Input: part model. Units: mm. Frame: model coordinates. Face numbers are marked on the shaded views. A direction names the side the tool comes from. Round coordinates to 2 decimals unless told otherwise and drop trailing zeros. Write each loop counter-clockwise with the first axis right and the second up, starting at its lowest first coordinate (ties: lowest second). Pieces come first, ordered by that corner, then holes. Notation, with made-up numbers: (9.25, 17) - (60.25, 17) arc R22 ccw to (60.25, 27) - close; hole circle Ø7 at (-7.5, -11.5). An arc over 180 degrees is marked (long way). Use one line per item in the form item = value.
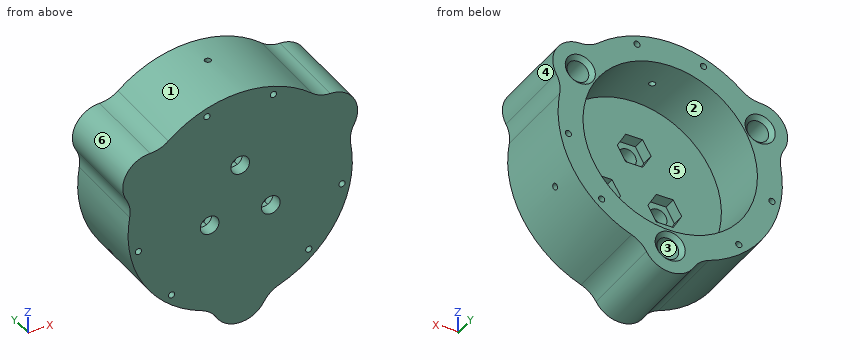
```python
from build123d import *

# Parameters (mm, degrees)
SKETCH_1_R               = 2.625
SKETCH_1_R_2             = 21
EXTRUDE_1_DEPTH          = 15
EXTRUDE_START            = 6
EXTRUDE_2_DEPTH          = 6
FILLET_1_R               = 7
CHAMFER_1_SIZE           = 1
SKETCH_4_R               = 2.25
CUT_EXTRUDE_1_DEPTH      = 48.335527685
CUT_EXTRUDE_2_DEPTH      = 3
SKETCH_6_R               = 0.75
CUT_EXTRUDE_3_DEPTH      = 48.335527685
SKETCH_7_R               = 0.75
CUT_EXTRUDE_4_DEPTH      = 45.996135167
PATTERN_CIRCULAR_1_COUNT = 3


with BuildPart() as part:
    # Эскиз1 → Бобышка-Вытянуть1 (new body)
    with BuildSketch(Plane(origin=(0, 0, 0), x_dir=(1, 0, 0), z_dir=(0, 1, 0))):
        with BuildLine():
            ThreePointArc((25.949265582, -7.458928593), (23.382685902, 13.5), (6.515011145, 26.2021875))
            ThreePointArc((6.515011145, 26.2021875), (0, 31.625), (-6.515011145, 26.2021875))
            ThreePointArc((-6.515011145, 26.2021875), (-23.382685902, 13.5), (-25.949265582, -7.458928593))
            ThreePointArc((-25.949265582, -7.458928593), (-27.388053395, -15.8125), (-19.434254437, -18.743258907))
            ThreePointArc((-19.434254437, -18.743258907), (0, -27), (19.434254437, -18.743258907))
            ThreePointArc((19.434254437, -18.743258907), (27.388053395, -15.8125), (25.949265582, -7.458928593))
        make_face()
        with Locations(Location((0, 25, 0), (0, 0, 270))):
            Circle(SKETCH_1_R, mode=Mode.SUBTRACT)
        with Locations(Location((0, 0, 0), (0, 0, 270))):
            Circle(SKETCH_1_R_2, mode=Mode.SUBTRACT)
        with Locations(Location((-21.650635095, -12.5, 0), (0, 0, 270))):
            Circle(SKETCH_1_R, mode=Mode.SUBTRACT)
        with Locations(Location((21.650635095, -12.5, 0), (0, 0, 270))):
            Circle(SKETCH_1_R, mode=Mode.SUBTRACT)
    extrude(amount=EXTRUDE_1_DEPTH)

    # Эскиз2 → Бобышка-Вытянуть2 (add)
    with BuildSketch(Plane.XZ.offset(EXTRUDE_START)):
        with BuildLine():
            ThreePointArc((25.949265582, 7.458928593), (27.388053395, 15.8125), (19.434254437, 18.743258907))
            ThreePointArc((19.434254437, 18.743258907), (0, 27), (-19.434254437, 18.743258907))
            ThreePointArc((-19.434254437, 18.743258907), (-27.388053395, 15.8125), (-25.949265582, 7.458928593))
            ThreePointArc((-25.949265582, 7.458928593), (-23.382685902, -13.5), (-6.515011145, -26.2021875))
            ThreePointArc((-6.515011145, -26.2021875), (0, -31.625), (6.515011145, -26.2021875))
            ThreePointArc((6.515011145, -26.2021875), (23.382685902, -13.5), (25.949265582, 7.458928593))
        make_face()
    extrude(amount=-EXTRUDE_2_DEPTH)

    # Скругление1
    fillet_1_edges = [part.edges().sort_by_distance(p)[0] for p in [
        (19.434254437, 4.5, 18.743258907),
        (-19.434254437, 4.5, 18.743258907),
        (-25.949265582, 4.5, 7.458928593),
        (-6.515011145, 4.5, -26.2021875),
        (6.515011145, 4.5, -26.2021875),
        (25.949265582, 4.5, 7.458928593),
    ]]
    fillet(fillet_1_edges, radius=FILLET_1_R)

    # Фаска1
    chamfer_1_edges = [part.edges().sort_by_distance(p)[0] for p in [
        (21.650635095, 15, 9.875),
        (0, 15, -27.625),
        (-21.650635095, 15, 9.875),
    ]]
    chamfer(chamfer_1_edges, length=CHAMFER_1_SIZE)

    # Эскиз4 → Вырез-Вытянуть1 (cut, through all)
    with BuildSketch(Plane.XZ.offset(6)):
        with Locations(Location((0, 8.5, 0), (0, 0, 270))):
            Circle(SKETCH_4_R)
        with Locations(Location((7.361215932, -4.25, 0), (0, 0, 270))):
            Circle(SKETCH_4_R)
        with Locations(Location((-7.361215932, -4.25, 0), (0, 0, 270))):
            Circle(SKETCH_4_R)
    extrude(amount=-CUT_EXTRUDE_1_DEPTH, mode=Mode.SUBTRACT)

    # Эскиз5 → Вырез-Вытянуть2 (cut)
    with BuildSketch(Plane(origin=(0, 0, 0), x_dir=(1, 0, 0), z_dir=(0, 1, 0))):
        Polygon((2.035159699, -12.025), (4.070319398, -8.5), (2.035159699, -4.975), (-2.035159699, -4.975), (-4.070319398, -8.5), (-2.035159699, -12.025), align=None)
        Polygon((5.326056233, 0.725), (9.396375631, 0.725), (11.43153533, 4.25), (9.396375631, 7.775), (5.326056233, 7.775), (3.290896534, 4.25), align=None)
        Polygon((-11.43153533, 4.25), (-9.396375631, 0.725), (-5.326056233, 0.725), (-3.290896534, 4.25), (-5.326056233, 7.775), (-9.396375631, 7.775), align=None)
    extrude(amount=-CUT_EXTRUDE_2_DEPTH, mode=Mode.SUBTRACT)

    # Эскиз6 → Вырез-Вытянуть3 (cut, through all)
    with BuildSketch(Plane(origin=(0, 15, 0), x_dir=(1, 0, 0), z_dir=(0, 1, 0))):
        with Locations(Location((-8, -23.685438565, 0), (0, 0, 270))):
            Circle(SKETCH_6_R)
        with Locations(Location((8, -23.685438565, 0), (0, 0, 270))):
            Circle(SKETCH_6_R)
        with Locations(Location((-16.512191497, 18.770922513, 0), (0, 0, 270))):
            Circle(SKETCH_6_R)
        with Locations(Location((-24.512191497, 4.914516052, 0), (0, 0, 270))):
            Circle(SKETCH_6_R)
        with Locations(Location((24.512191497, 4.914516052, 0), (0, 0, 270))):
            Circle(SKETCH_6_R)
        with Locations(Location((16.512191497, 18.770922513, 0), (0, 0, 270))):
            Circle(SKETCH_6_R)
    extrude(amount=-CUT_EXTRUDE_3_DEPTH, mode=Mode.SUBTRACT)

    # Эскиз7 → Вырез-Вытянуть4 (cut, through all)
    with BuildSketch(Plane.XY):
        with Locations(Location((0, 7.5, 0), (0, 0, 270.000000034))):
            Circle(SKETCH_7_R)
    cut_extrude_4 = extrude(amount=CUT_EXTRUDE_4_DEPTH, mode=Mode.SUBTRACT)

    # Круговой массив1: Вырез-Вытянуть4 ×3 about axis
    pattern_circular_1_axis = Axis((0, 15, 0), (0, -1, 0))
    for i in range(1, PATTERN_CIRCULAR_1_COUNT):
        add(cut_extrude_4.rotate(pattern_circular_1_axis, i * 360 / PATTERN_CIRCULAR_1_COUNT), mode=Mode.SUBTRACT)


solid = part.part
```
(1) Cut plane B-B on y = 7.5. Count the separate pieces of the cut face and the enclosed holes in it, then the cut area to 3 significant figures.
Derived:
separate_pieces = 3
enclosed_holes = 9
area = 948 mm^2
(2) Draft query along Z for the marked faces 1, 2, 3 and 4. Return one class per face: released by +Z, released by -Z, zero draft, split by the parting line, or undercut.
Derived:
face_1 = released by +Z
face_2 = undercut
face_3 = undercut
face_4 = split by the parting line
(3) Cut plane A-A on z = 0. Output: boundary loops of the cut face in (x, y).
Derived:
outline = (-27, -6) - (27, -6) - (27, 15) - (21, 15) - (21, 0) - (-21, 0) - (-21, 15) - (-27, 15) - close
(4) Material intervals for L1, parallel to X at y = -0.5, z = -1; L2, parallel to Z at x = -16.5, y = 11; L3, parallel to Z at x = 17, y = 3, sorted ascending.
Derived:
L1 = -26.98 to -9.56, -5.17 to 5.17, 9.56 to 26.98
L2 = -21.37 to -19.52, -18.02 to -12.99, 12.99 to 21.37
L3 = -20.98 to -19.34, -18.2 to -12.33, 12.33 to 20.98
(5) Access query for the marked faces 5 and 6. Directions: +Z, -Z, +X, -X, +Y, -Y. A direction counts if a zero-diameter tool reaches every point of the face in a straight line with its end or side. Return the directions, or none.
Derived:
face_5 = +Y
face_6 = -X, +Y, -Y
(6) First-contact query: pin 1 Ø10 at (x, y) = (19.5, 4) entering from +Z; pin 2 Ø8 at (x, y) = (15, -1.5) entering from -Z; pin 3 Ø1.5 at (x, y) = (11, 0) entering from -Z. Flat tips, straight axial feed; report the tip coordinate or a pass-through.
Derived:
pin_1 = 22.78
pin_2 = -24.66
pin_3 = -24.98
